from build123d import *

# Parameters (mm, degrees)
BOSS_EXTRUDE1_DEPTH         = 227.5
TAP_DRILL_FOR_M5X0_8_TAP1_D = 5
F_5_0_5_DIAMETER_HOLE1_D    = 5
SKETCH9_R                   = 1.5
CUT_EXTRUDE1_DEPTH          = 29


with BuildPart() as part:
    # Sketch1 → Boss-Extrude1 (new body)
    with BuildSketch(Plane.XY):
        Polygon((0, 5), (0, 0), (5, 0), (20, 0), (20, 5), (5, 5), (5, 20), (0, 20), align=None)
    extrude(amount=BOSS_EXTRUDE1_DEPTH)

    # Tap Drill for M5x0.8 Tap1 (through all)
    with Locations(Plane(origin=(0, 5, 0), x_dir=(1, 0, 0), z_dir=(0, 1, 0))):
        with Locations((12.5, -203.75), (12.5, -143.75), (12.5, -83.75), (12.5, -23.75)):
            Hole(TAP_DRILL_FOR_M5X0_8_TAP1_D / 2)

    # Ø5.0 (5) Diameter Hole1 (through all)
    with Locations(Plane(origin=(5, 0, 0), x_dir=(0, 0, -1), z_dir=(1, 0, 0))):
        with Locations((-177.5, 12.346163158), (-132.5, 12.346163158), (-95, 12.346163158), (-50, 12.346163158)):
            Hole(F_5_0_5_DIAMETER_HOLE1_D / 2)

    # Sketch9 → Cut-Extrude1 (cut)
    with BuildSketch(Plane.ZY):
        with Locations((33.704207464, 17.6675)):
            Circle(SKETCH9_R)
        with Locations((73.75, 17.6675)):
            Circle(SKETCH9_R)
        with Locations((113.75, 17.6675)):
            Circle(SKETCH9_R)
        with Locations((153.75, 17.6675)):
            Circle(SKETCH9_R)
        with Locations((193.75, 17.6675)):
            Circle(SKETCH9_R)
    extrude(amount=-CUT_EXTRUDE1_DEPTH, mode=Mode.SUBTRACT)


solid = part.part
The listing builds one solid part. Answer for the finished solid, in the listing's coordinates (mm). A direction names the side the tool comes from. Give positions to 0.01 mm unless a question says otherwise; leave off trailing zeros. Order: outer loops, then holes, each group sorted by start corner. A loop starts at its lowest first (then second) coordinate and runs counter-clockwise, first axis right, second up. Notation, with made-up numbers: (64, 11) -> (75, 11) arc R36 cw to (75, 50) -> close; hole circle Ø4 at (-36, 57). An arc over 180 degrees is marked (long way). Put each result on its own line as item: value.
Item 1: For a pull along X with two mould halves and no side action, classify faces 3 (the face through (0, 10, 112)), 4 (the face through (12.83, 2.47, 21.27)), 5 (the face through (5, 3, 0)), 6 (the face through (12.83, 2.47, 141.27)) as released by +X, released by -X, zero draft, split by the parting line, or undercut.
Established:
face 3: released by -X
face 4: undercut
face 5: zero draft
face 6: undercut
Item 2: A cutting plane is placed at C-C on x = 18. Give the vertices of the cut face in (y, z).
Established:
outline: (0, 0) -> (5, 0) -> (5, 227.5) -> (0, 227.5) -> close
Item 3: For faces 1 (the face through (14.998, 2.465, 83.64)), 2 (the face through (13, 5, 112)), determine the directions among +Z, -Z, +X, -X, +Y, -Y from which every point of the face is accessible in a straight line to the end or side of a thin tool.
Established:
face 1: +Y, -Y
face 2: +Z, -Z, +X, +Y
Item 4: Given P1, Ø3, axis at x = 7.5, z = 90.5, coming from the -Y side; P2, Ø4, axis at x = 12.5, z = 203.75, coming from the -Y side; P3, Ø3, axis at y = 7.5, z = 35.5, coming from the +X side; P4, Ø6, axis at x = 12.5, z = 23.75, coming from the +Y side, each flat-ended and moving along its own axis, determine where each tip first touches the part or whether it passes through.
Established:
P1: stops at y = 0
P2: passes through
P3: stops at x = 5
P4: stops at y = 5
Item 5: A cutting plane is placed at B-B on z = 60. Give the vertices of the cut face in (x, y), plus the area to 3 significant figures.
Established:
outline: (0, 0) -> (20, 0) -> (20, 5) -> (5, 5) -> (5, 20) -> (0, 20) -> close
area: 175 mm^2
Item 6: Straight lines are drawn through the part: line 1 (Z direction, x = 12.5, y = 3.3); line 2 (Y direction, x = 2, z = 95); line 3 (Y direction, x = 13, z = 103.5). For each, find the intervals that lie inside material, in ascending order.
Established:
line 1: z = 0 to 21.25, 26.25 to 81.25, 86.25 to 141.25, 146.25 to 201.25, 206.25 to 227.5
line 2: y = 0 to 9.85, 14.85 to 20
line 3: y = 0 to 5
Item 7: A cutting plane is placed at A-A on z = 83.75. Give the vertices of the cut face in (x, y), plus the area to 3 significant figures.
Established:
outline: (0, 0) -> (10, 0) -> (10, 5) -> (5, 5) -> (5, 20) -> (0, 20) -> close; (15, 0) -> (20, 0) -> (20, 5) -> (15, 5) -> close
area: 150 mm^2
